from build123d import *

# Parameters (mm, degrees)
BOSS_EXTRUDE1_DEPTH            = 70
BOSS_EXTRUDE2_DEPTH            = 70
CUT_EXTRUDE1_DEPTH             = 60
SKETCH13_W                     = 9
SKETCH13_H                     = 60
CUT_EXTRUDE3_DEPTH             = 5
SKETCH12_W                     = 25
SKETCH12_H                     = 23
CUT_EXTRUDE2_DEPTH             = 5
BOSS_EXTRUDE3_DEPTH            = 3.84
CBORE_FOR_M3_SHCS1_D           = 3.4
CBORE_FOR_M3_SHCS1_DEPTH       = 8.05
CBORE_FOR_M3_SHCS1_CBORE_D     = 6.5
CBORE_FOR_M3_SHCS1_CBORE_DEPTH = 4
CBORE_FOR_M3_SHCS1_TIP         = 1.021463052
M3X0_5_TAPPED_HOLE1_D          = 2.5
M3X0_5_TAPPED_HOLE1_DEPTH      = 14
M3X0_5_TAPPED_HOLE1_TIP        = 0.751075774
FILLET1_R                      = 10
FILLET4_R                      = 5
FILLET5_R                      = 3


with BuildPart() as part:
    # Sketch3 → Boss-Extrude1 (new body)
    with BuildSketch(Plane.XY):
        with BuildLine():
            Line((85.25, 15), (85.25, 40))
            Line((85.25, 40), (90.25, 40))
            Line((90.25, 40), (90.25, 15))
            ThreePointArc((90.25, 15), (84.392135624, 0.857864376), (70.25, -5))
            Line((70.25, -5), (-12, -5))
            Line((-12, -5), (-12, 60.2))
            Line((-12, 60.2), (0, 60.2))
            Line((0, 60.2), (0, 0))
            Line((0, 0), (70.25, 0))
            ThreePointArc((70.25, 0), (80.856601718, 4.393398282), (85.25, 15))
        make_face()
    extrude(amount=BOSS_EXTRUDE1_DEPTH)

    # Sketch5 → Boss-Extrude2 (add)
    with BuildSketch(Plane.XY.offset(70)):
        with BuildLine():
            Line((82.2, 15), (82.2, 40))
            Line((82.2, 40), (90.25, 40))
            Line((90.25, 40), (90.25, 15))
            ThreePointArc((90.25, 15), (84.392135624, 0.857864376), (70.25, -5))
            Line((70.25, -5), (25.1, -5))
            Line((25.1, -5), (25.1, 40))
            Line((25.1, 40), (33.15, 40))
            Line((33.15, 40), (33.15, 3.05))
            Line((33.15, 3.05), (70.25, 3.05))
            ThreePointArc((70.25, 3.05), (78.699926035, 6.550073965), (82.2, 15))
        make_face()
    extrude(amount=BOSS_EXTRUDE2_DEPTH)

    # Sketch6 → Cut-Extrude1 (cut)
    with BuildSketch(Plane.XY.offset(70)):
        Polygon((-3, 24.26), (0, 26.24), (0, 60.2), (-3, 60.2), align=None)
    extrude(amount=-CUT_EXTRUDE1_DEPTH, mode=Mode.SUBTRACT)

    # Sketch13 → Cut-Extrude3 (cut)
    with BuildSketch(Plane(origin=(0, 60.2, 0), x_dir=(1, 0, 0), z_dir=(0, 1, 0))):
        with Locations((-7.5, -40)):
            Rectangle(SKETCH13_W, SKETCH13_H)
    extrude(amount=-CUT_EXTRUDE3_DEPTH, mode=Mode.SUBTRACT)

    # Sketch12 → Cut-Extrude2 (cut)
    with BuildSketch(Plane(origin=(90.25, 0, 0), x_dir=(0, 0, -1), z_dir=(1, 0, 0))):
        with Locations((-50, 28.5)):
            Rectangle(SKETCH12_W, SKETCH12_H)
    extrude(amount=-CUT_EXTRUDE2_DEPTH, mode=Mode.SUBTRACT)

    # Sketch7 → Boss-Extrude3 (add)
    with BuildSketch(Plane.XY):
        with BuildLine():
            Line((-12, 60.2), (-12, -5))
            Line((-12, -5), (70.25, -5))
            ThreePointArc((70.25, -5), (84.392135624, 0.857864376), (90.25, 15))
            Line((90.25, 15), (90.25, 60.2))
            Line((90.25, 60.2), (-12, 60.2))
        make_face()
        with BuildLine():
            Line((70, 51.37), (40, 51.37))
            ThreePointArc((40, 51.37), (32.928932188, 48.441067812), (30, 41.37))
            Line((30, 41.37), (30, 11.37))
            ThreePointArc((30, 11.37), (32.928932188, 4.298932188), (40, 1.37))
            Line((40, 1.37), (70, 1.37))
            ThreePointArc((70, 1.37), (77.071067812, 4.298932188), (80, 11.37))
            Line((80, 11.37), (80, 41.37))
            ThreePointArc((80, 41.37), (77.071067812, 48.441067812), (70, 51.37))
        make_face(mode=Mode.SUBTRACT)
    extrude(amount=-BOSS_EXTRUDE3_DEPTH)

    # CBORE for M3 SHCS1
    with Locations(Plane(origin=(0, 3.05, 0), x_dir=(1, 0, 0), z_dir=(0, 1, 0))):
        with Locations((40.175, -82.5), (55.175, -82.5)):
            CounterBoreHole(CBORE_FOR_M3_SHCS1_D / 2, CBORE_FOR_M3_SHCS1_CBORE_D / 2, CBORE_FOR_M3_SHCS1_CBORE_DEPTH, depth=CBORE_FOR_M3_SHCS1_DEPTH)
            with Locations((0, 0, -(CBORE_FOR_M3_SHCS1_DEPTH + CBORE_FOR_M3_SHCS1_TIP / 2))):  # 118° drill point
                Cone(0, CBORE_FOR_M3_SHCS1_D / 2, CBORE_FOR_M3_SHCS1_TIP, mode=Mode.SUBTRACT)

    # M3x0.5 Tapped Hole1
    with Locations(Plane(origin=(0, 55.2, 0), x_dir=(1, 0, 0), z_dir=(0, 1, 0))):
        with Locations((-7.5, -25), (-7.5, -55)):
            Hole(M3X0_5_TAPPED_HOLE1_D / 2, depth=M3X0_5_TAPPED_HOLE1_DEPTH)
            with Locations((0, 0, -(M3X0_5_TAPPED_HOLE1_DEPTH + M3X0_5_TAPPED_HOLE1_TIP / 2))):  # 118° drill point
                Cone(0, M3X0_5_TAPPED_HOLE1_D / 2, M3X0_5_TAPPED_HOLE1_TIP, mode=Mode.SUBTRACT)

    # Fillet1
    fillet1_edges = [part.edges().sort_by_distance(p)[0] for p in [
        (25.1, -2.5, 70),
    ]]
    fillet(fillet1_edges, radius=FILLET1_R)

    # Fillet4
    fillet4_edges = [part.edges().sort_by_distance(p)[0] for p in [
        (87.75, 17, 37.5),
        (87.75, 17, 62.5),
    ]]
    fillet(fillet4_edges, radius=FILLET4_R)

    # Fillet5
    fillet5_edges = [part.edges().sort_by_distance(p)[0] for p in [
        (87.75, 40, 0),
        (90.25, 60.2, -1.92),
    ]]
    fillet(fillet5_edges, radius=FILLET5_R)


solid = part.part
Model file for the job. Use its own axes, mm. A direction names the side the tool comes from. Coordinates: 2 decimals unless noted, no trailing zeros. Write each loop counter-clockwise with the first axis right and the second up, starting at its lowest first coordinate (ties: lowest second). Pieces come first, ordered by that corner, then holes. Notation, with made-up numbers: (42.5, 33) -> (64.5, 33) arc R8 ccw to (64.5, 46) -> close; hole circle Ø5 at (41, 47.25). An arc over 180 degrees is marked (long way). One line per item, written item: value. Start each with the question number.
1) Slice it at A-A on z = 82.5. Write the cut outline in (x, y) (3 decimals), then the cut area to 3 significant figures.
2) Slice it at B-B on y = 35. Write the cut outline in (x, z), then the cut area to 3 significant figures.
3) Slice it at D-D on z = 17.5. Write the cut outline in (x, y), then the cut area to 3 significant figures.
4) Flat gauge pins, fed straight in: pin 1 Ø21 at (x, z) = (40.5, 37.5) entering from +Y; pin 2 Ø5.5 at (x, z) = (88, 28) entering from +Y; pin 3 Ø6 at (x, y) = (-8.5, 42) entering from +Z. Where does each tip first touch, or does it go through?
5) Slice it at C-C on x = 49.5. Write the cut outline in (y, z), then the cut area to 3 significant figures.
6) Pull direction X, two halves, no side cores. Call faces 1 (the face through (58.1, 2.8, 140)), 2 (the face through (56.675, 1.078, 85.383)), 3 (the face through (90.25, 26, 69)): +X half, -X half, draft (parallel to the pull), parting line (faces both ways), or undercut.
7) Probe probe 1 along X at (y, z) = (-3.1, 82.5) (3 decimals); probe 2 along X at (y, z) = (2.2, 82.5) (1 decimal); probe 3 along X at (y, z) = (36, 134.5). List the from-to ranges inside material, lowest first.
8) Which spindle directions (+Z, -Z, +X, -X, +Y, -Y) get a long thin tool onto all of the face, cutting with end or side? Do faces 4 (the face through (0, 17, 35)), 5 (the face through (89.39, 59.3, -1.95)), 6 (the face through (76.99, 4.22, -1.89)), 7 (the face through (80.74, 4.28, 34.51)), 8 (the face through (88, 17, 50)). Say none if no direction does.
Answers follow:
1. outline: (25.1, -5) -> (38.475, -5) -> (38.475, -0.95) -> (36.925, -0.95) -> (36.925, 3.05) -> (33.15, 3.05) -> (33.15, 40) -> (25.1, 40) -> close; (41.875, -5) -> (53.475, -5) -> (53.475, -0.95) -> (51.925, -0.95) -> (51.925, 3.05) -> (43.425, 3.05) -> (43.425, -0.95) -> (41.875, -0.95) -> close; (56.875, -5) -> (70.25, -5) arc R20 ccw to (90.25, 15) -> (90.25, 40) -> (82.2, 40) -> (82.2, 15) arc R11.95 cw to (70.25, 3.05) -> (58.425, 3.05) -> (58.425, -0.95) -> (56.875, -0.95) -> close
1. area: 985 mm2
2. outline: (-12, -3.84) -> (30, -3.84) -> (30, 0) -> (0, 0) -> (0, 10) -> (-3, 10) -> (-3, 70) -> (-12, 70) -> close; (25.1, 70) -> (33.15, 70) -> (33.15, 140) -> (25.1, 140) -> close; (80, -3.84) -> (90.25, -3.84) -> (90.25, 37.5) -> (85.25, 37.5) -> (85.25, 0) -> (80, 0) -> close; (82.2, 70) -> (85.25, 70) -> (85.25, 62.5) -> (90.25, 62.5) -> (90.25, 140) -> (82.2, 140) -> close
2. area: 2,210 mm2
3. outline: (-12, -5) -> (70.25, -5) arc R20 ccw to (90.25, 15) -> (90.25, 40) -> (85.25, 40) -> (85.25, 15) arc R15 cw to (70.25, 0) -> (0, 0) -> (0, 26.24) -> (-3, 24.26) -> (-3, 55.2) -> (-12, 55.2) -> close
3. area: 1,250 mm2
4. pin 1: y = 0
4. pin 2: y = 40
4. pin 3: z = 70
5. outline: (-5, -3.84) -> (1.37, -3.84) -> (1.37, 0) -> (0, 0) -> (0, 70) -> (3.05, 70) -> (3.05, 140) -> (-5, 140) -> close; (51.37, -3.84) -> (60.2, -3.84) -> (60.2, 0) -> (51.37, 0) -> close
5. area: 972 mm2
6. face 1: draft
6. face 2: undercut
6. face 3: +X half
7. probe 1: 25.1 to 38.475, 41.875 to 53.475, 56.875 to 78.758
7. probe 2: 25.1 to 36.9, 43.4 to 51.9, 58.4 to 85.6
7. probe 3: 25.1 to 33.15, 82.2 to 90.25
8. face 4: +Z, +Y
8. face 5: +Z, -Z, +X, +Y
8. face 6: -Z
8. face 7: +Y
8. face 8: +X, +Y
